```python
from build123d import *

# Parameters (mm, degrees)
F0_W     = 300
F0_H     = 24.5
F0_R     = 2.65
F1_DEPTH = 2
F2_DEPTH = 10
F3_DEPTH = 30
F4_R     = 1.7
F5_DEPTH = 2
F6_R     = 1.25
F7_DEPTH = 2


with BuildPart() as f1:
    # F0 (on Top) → F1 (new body)
    with BuildSketch(Plane.XY):
        Rectangle(F0_W, F0_H)
        with Locations((-90, 0)):
            Circle(F0_R, mode=Mode.SUBTRACT)
        with Locations((-75, 0)):
            Circle(F0_R, mode=Mode.SUBTRACT)
        with Locations((-60, 0)):
            Circle(F0_R, mode=Mode.SUBTRACT)
        with Locations((-45, 0)):
            Circle(F0_R, mode=Mode.SUBTRACT)
        with Locations((-30, 0)):
            Circle(F0_R, mode=Mode.SUBTRACT)
        with Locations((-15, 0)):
            Circle(F0_R, mode=Mode.SUBTRACT)
        Circle(F0_R, mode=Mode.SUBTRACT)
        with Locations((15, 0)):
            Circle(F0_R, mode=Mode.SUBTRACT)
        with Locations((30, 0)):
            Circle(F0_R, mode=Mode.SUBTRACT)
        with Locations((45, 0)):
            Circle(F0_R, mode=Mode.SUBTRACT)
        with Locations((60, 0)):
            Circle(F0_R, mode=Mode.SUBTRACT)
        with Locations((75, 0)):
            Circle(F0_R, mode=Mode.SUBTRACT)
        with Locations((90, 0)):
            Circle(F0_R, mode=Mode.SUBTRACT)
    extrude(amount=F1_DEPTH)

    # F2 (add): a face of the model
    f2_faces = [f1.faces().sort_by_distance(p)[0] for p in [
        (-150, 0, 1),
    ]]
    extrude(f2_faces, amount=F2_DEPTH)

    # F3 (add): a face of the model
    f3_faces = [f1.faces().sort_by_distance(p)[0] for p in [
        (150, 0, 1),
    ]]
    extrude(f3_faces, amount=F3_DEPTH)

    # F4 (on face) → F5 (cut, through all)
    with BuildSketch(Plane.XY.offset(2)):
        with Locations((-153.6, 0)):
            Circle(F4_R)
    extrude(amount=-F5_DEPTH, mode=Mode.SUBTRACT)

    # F6 (on face) → F7 (cut, through all)
    with BuildSketch(Plane.XY.offset(2)):
        with Locations((158.75, -7.25)):
            Circle(F6_R)
    extrude(amount=-F7_DEPTH, mode=Mode.SUBTRACT)


solid = f1.part
```
Could you check a few things on this model? Use its own coordinates, in mm. Give positions to 0.01 mm unless a question says otherwise; leave off trailing zeros.
Q1. We'd pull the mould along Y, two halves only. Please class faces 1 (the cylindrical face through (-12.472, 0.796, 0.986)), 2 (the flat face through (8, 0, 0)): +Y half, -Y half, draft (parallel to the pull), parting line (faces both ways), or undercut.
Q2. If I drill on line 1 along Y through (x, z) = (-15, 1.35); line 2 along X through (y, z) = (-7, 1.65); line 3 along Y through (x, z) = (-76.5, 1.45), over which ranges is the centre line in solid material (lowest first)?
Q3. Suppose I cut it at A-A, the plane z = 1. Count the separate pieces of the cut face and the enclosed holes in it, and give its area (3 significant figures).
Solution:
1. face 1: undercut
1. face 2: draft
2. line 1: y = -12.25 to -2.65, 2.65 to 12.25
2. line 2: x = -160 to 157.53, 159.97 to 180
2. line 3: y = -12.25 to -2.18, 2.18 to 12.25
3. separate pieces: 1
3. enclosed holes: 15
3. area: 8,030 mm2
